Could you check a few things on this model? Use its own coordinates, in mm. Give positions to 0.01 mm unless a question says otherwise; leave off trailing zeros. Write each loop counter-clockwise with the first axis right and the second up, starting at its lowest first coordinate (ties: lowest second). Pieces come first, ordered by that corner, then holes. Notation, with made-up numbers: M 14.25,61.25 L 58.25,61.25 A16 cw 58.25,85.25 Z; hole C -33.5,80.5 d7. An arc over 180 degrees is marked long. Use one line per item in the form item = value.
from build123d import *

# Parameters (mm, degrees)
BOSS_EXTRUDE1_DEPTH   = 1.2192
CHAMFER1_SIZE         = 5.08
CHAMFER1_SIZE2        = 1.0287
CHAMFER1_PART_2_SIZE  = 5.08
CHAMFER1_PART_2_SIZE2 = 1.0287
CHAMFER2_SIZE         = 5.08
CHAMFER2_SIZE2        = 1.0287
CHAMFER2_PART_2_SIZE  = 5.08
CHAMFER2_PART_2_SIZE2 = 1.0287


with BuildPart() as part:
    # Sketch1 → Boss-Extrude1 (new body, symmetric)
    with BuildSketch(Plane.XY):
        Polygon((0, 0), (101.6, 57.15), (127, 57.15), (133.35, 0), align=None)
    extrude(amount=BOSS_EXTRUDE1_DEPTH, both=True)

    # Chamfer1
    chamfer1_edges = [part.edges().sort_by_distance(p)[0] for p in [
        (50.8, 28.575, 1.2192),
    ]]
    chamfer1_side = [part.faces().sort_by_distance(p)[0] for p in [
        (85.09, 22.098, 1.2192),
    ]]
    chamfer(chamfer1_edges, length=CHAMFER1_SIZE, length2=CHAMFER1_SIZE2, reference=chamfer1_side[0])

    # Chamfer1 part 2
    chamfer1_part_2_edges = [part.edges().sort_by_distance(p)[0] for p in [
        (50.8, 28.575, -1.2192),
    ]]
    chamfer1_part_2_side = [part.faces().sort_by_distance(p)[0] for p in [
        (85.09, 22.098, -1.2192),
    ]]
    chamfer(chamfer1_part_2_edges, length=CHAMFER1_PART_2_SIZE, length2=CHAMFER1_PART_2_SIZE2, reference=chamfer1_part_2_side[0])

    # Chamfer2
    chamfer2_edges = [part.edges().sort_by_distance(p)[0] for p in [
        (130.175, 28.575, -1.2192),
    ]]
    chamfer2_side = [part.faces().sort_by_distance(p)[0] for p in [
        (89.460516254, 21.125525936, -1.2192),
    ]]
    chamfer(chamfer2_edges, length=CHAMFER2_SIZE, length2=CHAMFER2_SIZE2, reference=chamfer2_side[0])

    # Chamfer2 part 2
    chamfer2_part_2_edges = [part.edges().sort_by_distance(p)[0] for p in [
        (130.175, 28.575, 1.2192),
    ]]
    chamfer2_part_2_side = [part.faces().sort_by_distance(p)[0] for p in [
        (89.460516254, 21.125525936, 1.2192),
    ]]
    chamfer(chamfer2_part_2_edges, length=CHAMFER2_PART_2_SIZE, length2=CHAMFER2_PART_2_SIZE2, reference=chamfer2_part_2_side[0])


solid = part.part
1) For pin 1 Ø1 at (x, y) = (36, 20) entering from -Z, with a flat end and sliding along its axis, tell me the tip position at first contact or that it passes through.
Checked values:
pin_1 = -0.34
2) I want a section at C-C, the plane z = 0.7. Please give me the cut outline in (x, y), plus the area to 3 significant figures.
Checked values:
outline = M 5.13,0 L 130.82,0 L 124.47,57.15 L 106.73,57.15 Z
area = 4,100 mm2
3) I want a section at D-D, the plane y = 22. Please give me the cut outline in (x, z), plus the area to 3 significant figures.
Checked values:
outline = M 39.11,-0.19 L 49.47,-1.22 L 125.79,-1.22 L 130.91,-0.19 L 130.91,0.19 L 125.79,1.22 L 49.47,1.22 L 39.11,0.19 Z
area = 208 mm2
4) If I drill on L1, parallel to Y at x = 11, z = 0.05; L2, parallel to Z at x = 123, y = 54.5; L3, parallel to X at y = 4, z = -0.1, over which ranges is the centre line in solid material (lowest first)?
Checked values:
L1 = 0 to 6.19
L2 = -1.05 to 1.05
L3 = 7.11 to 132.91
5) I want a section at A-A, the plane y = 39.5. Please give me the cut outline in (x, z).
Checked values:
outline = M 70.22,-0.19 L 80.58,-1.22 L 123.85,-1.22 L 128.96,-0.19 L 128.96,0.19 L 123.85,1.22 L 80.58,1.22 L 70.22,0.19 Z
6) I want a section at B-B, the plane x = 87. Please give me the cut outline in (y, z).
Checked values:
outline = M 0,-1.22 L 43.11,-1.22 L 48.94,-0.19 L 48.94,0.19 L 43.11,1.22 L 0,1.22 Z
